Check sheet for the modelled part. Datum: model origin and axes. Units: mm. Face numbers are marked on the shaded views. A direction names the side the tool comes from. Give positions to 0.01 mm unless a question says otherwise; leave off trailing zeros. Loops run counter-clockwise (first coordinate to the right, second up) from the corner with the lowest first, then second, coordinate; pieces in that order, holes last. Notation, with made-up numbers: (55.25, 66) -> (110.25, 66) arc R18 ccw to (110.25, 75) -> close; hole circle Ø1 at (36, -35). An arc over 180 degrees is marked (long way). Write each question's results on one line, items separated by ' | '. Start each with the question number.
1. Tool access check on the marked faces 4, 5 and 6. Record the directions out of +Z, -Z, +X, -X, +Y, -Y that give a thin tool (end or side, any length) a straight path to the whole face; none if there is none.
2. Cross-section at C-C on y = -1.25. Record the boundary of the cut face in (x, z), and give its area (3 significant figures).
3. Cross-section at B-B on z = 35.5. Record the boundary of the cut face in (x, y).
4. Cross-section at A-A on x = 0. Record the boundary of the cut face in (y, z) (3 decimals), and give its area (4 significant figures).
5. Mould release check, pull along Z, two halves, no side actions. Record for the marked faces 1, 2 and 3: +Z half, -Z half, draft (parallel to the pull), parting line (faces both ways), or undercut.
6. Material ranges on L1, parallel to Z at x = 0, y = -4.25 (3 decimals); L2, parallel to X at y = -4.25, z = 22.5; L3, parallel to Z at x = 14.5, y = -5.5, recorded low to high. Write a range as from..to.
7. Cross-section at D-D on z = 40. Record the boundary of the cut face in (x, y).
8. Gauge pin test, flat ends, axial feed: pin 1 Ø1 at (y, z) = (-1.5, 11) entering from -X; pin 2 Ø5.5 at (x, z) = (-2, 10.5) entering from +Y; pin 3 Ø0.9 at (x, z) = (0, 9.5) entering from -Y; pin 4 Ø1.5 at (x, y) = (3.5, -6.5) entering from -Z. Record the tip position at first contact, or that the pin passes through.
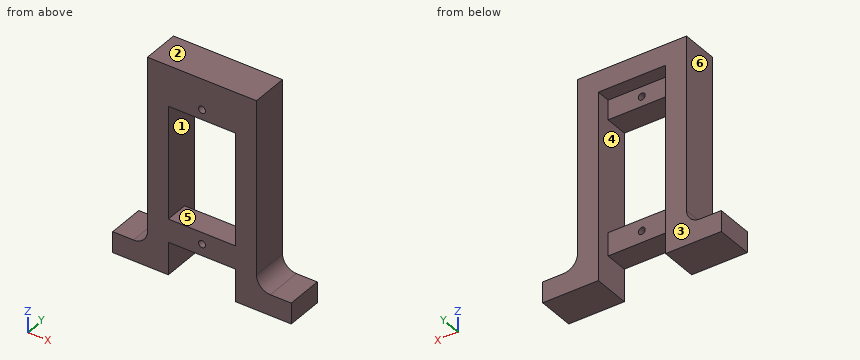
from build123d import *

# Parameters (mm, degrees)
F1_DEPTH = 8
F2_W     = 14.5
F2_H     = 4.25
F2_H_2   = 5
F3_DEPTH = 5
F4_R     = 0.75
F5_DEPTH = 5.001


with BuildPart() as f1:
    # F0 (on Front) → F1 (new body)
    with BuildSketch(Plane.XZ):
        with BuildLine():
            Line((-19.25, 4.5), (-19.25, 0))
            Line((-19.25, 0), (-7.25, 0))
            Line((-7.25, 0), (-7.25, 40.5))
            Line((-7.25, 40.5), (7.25, 40.5))
            Line((7.25, 40.5), (7.25, 0))
            Line((7.25, 0), (19.25, 0))
            Line((19.25, 0), (19.25, 4.5))
            Line((19.25, 4.5), (14.75, 4.5))
            ThreePointArc((14.75, 4.5), (12.62868, 5.37868), (11.75, 7.5))
            Line((11.75, 7.5), (11.75, 45))
            Line((11.75, 45), (-11.75, 45))
            Line((-11.75, 45), (-11.75, 7.5))
            ThreePointArc((-11.75, 7.5), (-12.62868, 5.37868), (-14.75, 4.5))
            Line((-14.75, 4.5), (-19.25, 4.5))
        make_face()
    extrude(amount=F1_DEPTH)

    # F2 (on face) → F3 (join)
    with BuildSketch(Plane.XZ.offset(8)):
        with Locations((0, 38.375)):
            Rectangle(F2_W, F2_H)
        with Locations((0, 9.5)):
            Rectangle(F2_W, F2_H_2)
    extrude(amount=-F3_DEPTH)

    # F4 (on face) → F5 (cut, through all)
    with BuildSketch(Plane(origin=(0, -3, 0), x_dir=(-1, 0, 0), z_dir=(0, 1, 0))):
        with Locations((0, 38.375)):
            Circle(F4_R)
        with Locations((0, 9.5)):
            Circle(F4_R)
    extrude(amount=-F5_DEPTH, mode=Mode.SUBTRACT)


solid = f1.part
Geometry says:
1) face 4: +Y | face 5: +Y, -Y | face 6: +Z, -X, +Y, -Y
2) outline: (-19.25, 0) -> (-7.25, 0) -> (-7.25, 40.5) -> (7.25, 40.5) -> (7.25, 0) -> (19.25, 0) -> (19.25, 4.5) -> (14.75, 4.5) arc R3 cw to (11.75, 7.5) -> (11.75, 45) -> (-11.75, 45) -> (-11.75, 7.5) arc R3 cw to (-14.75, 4.5) -> (-19.25, 4.5) -> close | area: 542 mm^2
3) outline: (-11.75, -8) -> (-7.25, -8) -> (-7.25, 0) -> (-11.75, 0) -> close; (7.25, -8) -> (11.75, -8) -> (11.75, 0) -> (7.25, 0) -> close
4) outline: (-8, 7) -> (-3, 7) -> (-3, 8.75) -> (-8, 8.75) -> close; (-8, 10.25) -> (-3, 10.25) -> (-3, 12) -> (-8, 12) -> close; (-8, 36.25) -> (-3, 36.25) -> (-3, 37.625) -> (-8, 37.625) -> close; (-8, 39.125) -> (-3, 39.125) -> (-3, 40.5) -> (0, 40.5) -> (0, 45) -> (-8, 45) -> close | area: 67.25 mm^2
5) face 1: undercut | face 2: +Z half | face 3: draft
6) L1: 7..8.75, 10.25..12, 36.25..37.625, 39.125..45 | L2: -11.75..-7.25, 7.25..11.75 | L3: 0..4.51
7) outline: (-11.75, -8) -> (11.75, -8) -> (11.75, 0) -> (7.25, 0) -> (7.25, -3) -> (-7.25, -3) -> (-7.25, 0) -> (-11.75, 0) -> close
8) pin 1: x = -11.75 | pin 2: y = -3 | pin 3: through | pin 4: z = 7
